Here's how the part is built. I have some questions about the finished solid (model axes, mm). A direction names the side the tool comes from. Round coordinates to 2 decimals unless told otherwise and drop trailing zeros. Order: outer loops, then holes, each group sorted by start corner. A loop starts at its lowest first (then second) coordinate and runs counter-clockwise, first axis right, second up. Notation, with made-up numbers: (-13, 48.25) - (19, 48.25) arc R27 ccw to (19, 74.25) - close; hole circle Ø3 at (3, -12). An arc over 180 degrees is marked (long way). Answer as a JSON object with one key per item and string values.
```python
from build123d import *

# Parameters (mm, degrees)
BOSS_EXTRUDE1_DEPTH = 3


with BuildPart() as part:
    # Sketch1 → Boss-Extrude1 (new body)
    with BuildSketch(Plane.XY):
        Polygon((-15, -15), (15, 20), (-15, 20), (-15, 7.5), (-18, 7.5), (-18, -7.5), (-15, -7.5), align=None)
        Polygon((1.724708718, 14.5), (4.002478525, 12.54762588), (-5.759392077, 1.158776844), (-8.037161884, 3.111150965), align=None, mode=Mode.SUBTRACT)
    extrude(amount=BOSS_EXTRUDE1_DEPTH)


solid = part.part
```
1. For faces 4 (the face through (-6.88, 2.12, 1.48)), 5 (the face through (-15, -11, 1)), 6 (the face through (-18, 0, 1)), which set-ups out of +Z, -Z, +X, -X, +Y, -Y let a thin tool reach every point of the face, with its end or its side?
Responses:
{"face 4": "+Z, -Z", "face 5": "+Z, -Z, -X, -Y", "face 6": "+Z, -Z, -X, +Y, -Y"}
2. Imagine slicing it at D-D (x = 13.5). List the corners of the cut face in (y, z) for me.
Responses:
{"outline": "(18.25, 0) - (20, 0) - (20, 3) - (18.25, 3) - close"}
3. Imagine slicing it at C-C (x = -4.5). List the corners of the cut face in (y, z) for me.
Responses:
{"outline": "(-2.75, 0) - (2.63, 0) - (2.63, 3) - (-2.75, 3) - close; (7.24, 0) - (20, 0) - (20, 3) - (7.24, 3) - close"}
4. Imagine slicing it at A-A (z = 0.9). List the corners of the cut face in (x, y) for me, plus the area to 3 significant figures.
Responses:
{"outline": "(-18, -7.5) - (-15, -7.5) - (-15, -15) - (15, 20) - (-15, 20) - (-15, 7.5) - (-18, 7.5) - close; hole (-8.04, 3.11) - (-5.76, 1.16) - (4, 12.55) - (1.72, 14.5) - close", "area": "525 mm2"}
5. Thinking about a two-plate mould opening in Y: for faces 1 (the face through (-16, 7.5, 1)), 2 (the face through (-0.81, 6.93, 1.48)), 3 (the face through (-15, 14, 1)), which applies, pulls with the +Y half, pulls with the -Y half, needs draft (parallel to the pull), parting line crosses it, or undercut?
Responses:
{"face 1": "pulls with the +Y half", "face 2": "undercut", "face 3": "needs draft"}
6. If I drill on L1, parallel to Y at x = -2.5, z = 0.2; L2, parallel to X at y = 7, z = 0.2; L3, parallel to X at y = 4.5, z = 1.25, over which ranges is the centre line in solid material (lowest first)? Write a range as [from, to].
Responses:
{"L1": "[-0.42, 4.96], [9.57, 20]", "L2": "[-18, -4.7], [-0.75, 3.86]", "L3": "[-18, -6.85], [-2.9, 1.71]"}
7. Imagine slicing it at B-B (y = 5.5). List the corners of the cut face in (x, z) for me.
Responses:
{"outline": "(-18, 0) - (-5.99, 0) - (-5.99, 3) - (-18, 3) - close; (-2.04, 0) - (2.57, 0) - (2.57, 3) - (-2.04, 3) - close"}
8. For P1, Ø1.5, axis at x = -17, z = 2, coming from the +Y side; P2, Ø1.5, axis at x = -17, z = 1.5, coming from the -Y side; P3, Ø4, axis at x = -6.5, y = 6.5, coming from the -Z side; P4, Ø0.9, axis at y = -10.5, z = 2, coming from the -X side, each with a flat end and sliding along its axis, tell me the tip position at first contact or that it passes through.
Responses:
{"P1": "y = 7.5", "P2": "y = -7.5", "P3": "z = 0", "P4": "x = -15"}
